```python
from build123d import *

# Parameters (mm, degrees)
F1_DEPTH     = 12.5
F3_DEPTH     = 145
F4_W         = 200
F4_H         = 19
F5_DEPTH     = 5
F7_DEPTH     = 5
F8_R         = 1
F9_DEPTH     = 135.4900855741
F11_T3_ANGLE = 288.8835060345
F11_T7_ANGLE = 288.8835060345
F12_W        = 164.3678992987
F12_H        = 299.086984247
F13_DEPTH    = 15
F14_R        = 1.5
F15_DEPTH    = 3
F16_R        = 1.5
F17_DEPTH    = 3
F18_SIZE     = 0.5
F19_R        = 1.5
F20_DEPTH    = 134.5119145259
F21_R        = 7


# Not quite as in the source:
# - a fillet or chamfer that OpenCascade refuses, or shapes differently, is made with other operations: its cross-section is extruded or revolved along the edge and cut away or added


with BuildPart() as f1:
    # F0 (on Front) → F1 (new body, symmetric)
    with BuildSketch(Plane.XZ):
        with BuildLine():
            ThreePointArc((95.206740787, 0), (-0.4890855741, 230.2224176182), (-96.1849119353, 0))
            Line((-96.1849119353, 0), (95.206740787, 0))
        make_face()
    extrude(amount=F1_DEPTH, both=True)

    # F2 (on face) → F3 (cut, symmetric)
    with BuildSketch(Plane.XZ.offset(12.5)):
        with BuildLine():
            ThreePointArc((80.206740787, 0), (-0.4890855741, 220.4629960136), (-81.1849119353, 0))
            Line((-81.1849119353, 0), (80.206740787, 0))
        make_face()
    extrude(amount=F3_DEPTH, both=True, mode=Mode.SUBTRACT)

    # F4 (on Top) → F5 (join)
    with BuildSketch(Plane.XY):
        Rectangle(F4_W, F4_H)
    extrude(amount=-F5_DEPTH)

    # F6 (on Front) → F7 (cut, symmetric)
    with BuildSketch(Plane.XZ):
        with BuildLine():
            ThreePointArc((86.5775826458, -1.0740190898), (-0.4890855741, 225.4629960136), (-87.5557537941, -1.0740190898))
            Line((-87.5557537941, -1.0740190898), (86.5775826458, -1.0740190898))
        make_face()
    extrude(amount=F7_DEPTH, both=True, mode=Mode.SUBTRACT)

    # F8 (on Right) → F9 (cut, through all)
    with BuildSketch(Plane.YZ):
        Circle(F8_R)
    extrude(amount=-F9_DEPTH, mode=Mode.SUBTRACT)

    # F11: fillet of radius 9 on 2 edges, made by hand


with BuildPart() as f11_tool1:
    # F11_s2 → F11_t3 (revolve)
    with BuildSketch(Plane(origin=(44.7250174756, 0, 31.9706955431), x_dir=(0, 1, 0), z_dir=(-0.8135247542, 0, -0.5815302867))):
        with BuildLine():
            ThreePointArc((-12.5, 48.2497880385), (-9.8639610307, 54.6137490692), (-3.5, 57.2497880385))
            Line((-3.5, 57.2497880385), (-3.5, 57.4297880385))
            Line((-3.5, 57.4297880385), (-12.68, 57.4297880385))
            Line((-12.68, 57.4297880385), (-12.68, 48.2497880385))
            Line((-12.68, 48.2497880385), (-12.5, 48.2497880385))
        make_face()
    revolve(axis=Axis((-0.4890855741, -12.5, 95.2224176182), (0, -1, 0)), revolution_arc=F11_T3_ANGLE)

    split(bisect_by=Plane.XY, keep=Keep.TOP)


with BuildPart() as f11_tool5:
    # F11_s6 → F11_t7 (revolve)
    with BuildSketch(Plane(origin=(44.7250174756, 0, 31.9706955431), x_dir=(0, 1, 0), z_dir=(-0.8135247542, 0, -0.5815302867))):
        with BuildLine():
            ThreePointArc((3.5, 57.2497880385), (9.8639610307, 54.6137490692), (12.5, 48.2497880385))
            Line((12.5, 48.2497880385), (12.68, 48.2497880385))
            Line((12.68, 48.2497880385), (12.68, 57.4297880385))
            Line((12.68, 57.4297880385), (3.5, 57.4297880385))
            Line((3.5, 57.4297880385), (3.5, 57.2497880385))
        make_face()
    revolve(axis=Axis((-0.4890855741, 12.5, 95.2224176182), (0, -1, 0)), revolution_arc=F11_T7_ANGLE)

    split(bisect_by=Plane.XY, keep=Keep.TOP)


with BuildPart() as f1_1:
    add(f1.part)

    # F11_t9: cut F11_tool1, F11_tool5
    add([f11_tool1.part, f11_tool5.part], mode=Mode.SUBTRACT)

    # F12 (on Front) → F13 (cut, symmetric)
    with BuildSketch(Plane.XZ):
        with Locations((-82.1839496493, 121.752621606)):
            Rectangle(F12_W, F12_H)
    extrude(amount=F13_DEPTH, both=True, mode=Mode.SUBTRACT)

    # F14 (on face) → F15 (join)
    with BuildSketch(Plane(origin=(0, 0, 0), x_dir=(0, -1, 0), z_dir=(-1, 0, 0))):
        with Locations((-8.75, 225.4620759923)):
            Circle(F14_R)
    extrude(amount=F15_DEPTH)

    # F16 (on face) → F17 (cut)
    with BuildSketch(Plane(origin=(0, 0, 0), x_dir=(0, -1, 0), z_dir=(-1, 0, 0))):
        with Locations((8.75, 225.4620759923)):
            Circle(F16_R)
    extrude(amount=-F17_DEPTH, mode=Mode.SUBTRACT)

    # F18
    f18_edges = [f1_1.edges().sort_by_distance(p)[0] for p in [
        (-3, 10.25, 225.462076),
    ]]
    chamfer(f18_edges, length=F18_SIZE)

    # F19 (on Right) → F20 (cut, through all)
    with BuildSketch(Plane.YZ):
        Circle(F19_R)
    extrude(amount=F20_DEPTH, mode=Mode.SUBTRACT)

    # F21
    f21_edges = [f1_1.edges().sort_by_distance(p)[0] for p in [
        (100, 9.5, -2.5),
        (100, -9.5, -2.5),
    ]]
    fillet(f21_edges, radius=F21_R)


solid = f1_1.part
```
Build history of the part. All positions in model axes, mm. A direction names the side the tool comes from. Give positions to 0.01 mm unless a question says otherwise; leave off trailing zeros.
1) Probe line 1 along Z through (x, y) = (2.3, -8.75); line 2 along Z through (x, y) = (54.5, 2); line 3 along Z through (x, y) = (89, 1.25). List the from-to ranges inside material, lowest first.
Values follow:
line 1: z = -5 to 0, 220.43 to 223.96, 226.96 to 228.5
line 2: z = -5 to -1.07, 213.26 to 218.52
line 3: z = -5 to -0.83, 0.83 to 1.17, 189.76 to 196.3
2) Drop flat-ended pins along their axis: P1, Ø2.5, axis at y = -3, z = -2.5, coming from the -X side; P2, Ø12, axis at y = 9.5, z = 76, coming from the -X side; P3, Ø3, axis at x = 25, y = 4, coming from the +Z side. Give the stop position or say it passes through.
Values follow:
P1: stops at x = 0
P2: stops at x = 121.89
P3: stops at z = 228.07
3) 3-axis set-ups, long thin cutter, end or side, ignore diameter. For faces 1 (the face through (40, -7, 0)), 2 (the face through (100, 0, -3)), 3 (the face through (46, -9.5, -2)), 4 (the face through (117, 5, 146)): which of +Z, -Z, +X, -X, +Y, -Y reach the whole face in a straight line?
Values follow:
face 1: -X, +Y, -Y
face 2: -Z, +X, +Y, -Y
face 3: -Z, +X, -X, -Y
face 4: -X
4) Two-plate mould, pull along Y, no slides. Class faces 5 (the face through (97.9, 7.5, -2.5)), 6 (the face through (0, 0, -3)), 7 (the face through (121.71, -0.07, 139.82)): released by +Y, released by -Y, zero draft, split by the parting line, or undercut.
Values follow:
face 5: released by +Y
face 6: zero draft
face 7: undercut
